Read the model definition and answer for the solid it produces. Units are mm, in the model's axes. Give positions to 0.01 mm unless a question says otherwise; leave off trailing zeros. Loops run counter-clockwise (first coordinate to the right, second up) from the corner with the lowest first, then second, coordinate; pieces in that order, holes last.
(1) Each of these flat-tipped pins is pushed along its axis until it touches: P1, Ø5.5, axis at x = -29.18, y = 15.5, coming from the -Z side; P2, Ø4.5, axis at x = 29.18, y = 15.5, coming from the -Z side. Where does it stop, or does it pass through?
(2) Find section B-B, the plane z = 0.8. Write down the section's boundary in (x, y).
(3) Straight lines are drawn through the part: probe 1 along X at (y, z) = (-15.5, 2.75); probe 2 along X at (y, z) = (16, 0.5). For each, find the intervals that lie inside material, in ascending order.
(4) Find section A-A, the plane y = 15.5. Write down the section's boundary in (x, z) (3 decimals), then the cut area to 3 significant figures.
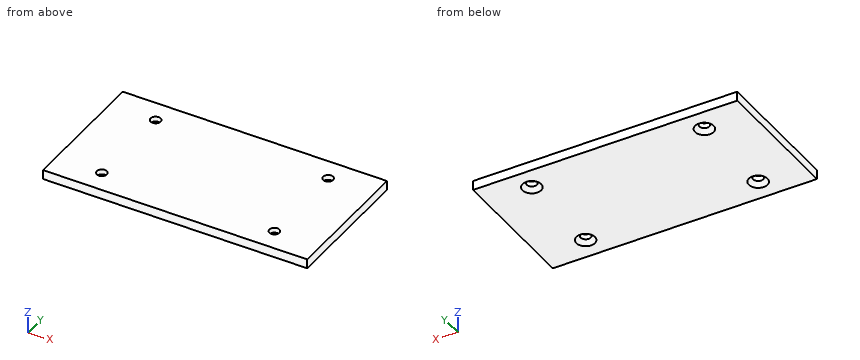
```python
from build123d import *

# Parameters (mm, degrees)
PROFILE_SKETCH_W                                = 89.349072
PROFILE_SKETCH_H                                = 46
PROFILE_EXTRUDE_DEPTH                           = 3.175
CSK_FOR_M3_FLAT_HEAD_MACHINE_SCREW1_D           = 3.4
CSK_FOR_M3_FLAT_HEAD_MACHINE_SCREW1_CSINK_D     = 6.3
CSK_FOR_M3_FLAT_HEAD_MACHINE_SCREW1_CSINK_ANGLE = 90


with BuildPart() as part:
    # Profile Sketch → Profile Extrude (new body)
    with BuildSketch(Plane.XY):
        Rectangle(PROFILE_SKETCH_W, PROFILE_SKETCH_H)
    extrude(amount=PROFILE_EXTRUDE_DEPTH)

    # CSK for M3 Flat Head Machine Screw1 (through all)
    with Locations(Plane(origin=(-29.175456, 15.500000014, 0), x_dir=(-1, 0, 0), z_dir=(0, 0, -1))):
        with Locations((0, 0), (0, -31.000000028), (-58.350912, -31.000000028), (-58.350912, 0)):
            CounterSinkHole(CSK_FOR_M3_FLAT_HEAD_MACHINE_SCREW1_D / 2, CSK_FOR_M3_FLAT_HEAD_MACHINE_SCREW1_CSINK_D / 2, counter_sink_angle=CSK_FOR_M3_FLAT_HEAD_MACHINE_SCREW1_CSINK_ANGLE)


solid = part.part
```
Entries:
1. P1: stops at z = 0.4
1. P2: stops at z = 0.9
2. outline: (-44.67, -23) - (44.67, -23) - (44.67, 23) - (-44.67, 23) - close; hole circle Ø4.7 at (-29.18, -15.5); hole circle Ø4.7 at (-29.18, 15.5); hole circle Ø4.7 at (29.18, -15.5); hole circle Ø4.7 at (29.18, 15.5)
3. probe 1: x = -44.67 to -30.88, -27.48 to 27.48, 30.88 to 44.67
3. probe 2: x = -44.67 to -31.78, -26.57 to 26.57, 31.78 to 44.67
4. outline: (-44.675, 0) - (-32.325, 0) - (-30.875, 1.45) - (-30.875, 3.175) - (-44.675, 3.175) - close; (-27.475, 1.45) - (-26.025, 0) - (26.025, 0) - (27.475, 1.45) - (27.475, 3.175) - (-27.475, 3.175) - close; (30.875, 1.45) - (32.325, 0) - (44.675, 0) - (44.675, 3.175) - (30.875, 3.175) - close
4. area: 258 mm2
